Build history of the part. All positions in model axes, mm. A direction names the side the tool comes from. Give positions to 0.01 mm unless a question says otherwise; leave off trailing zeros. Write each loop counter-clockwise with the first axis right and the second up, starting at its lowest first coordinate (ties: lowest second). Pieces come first, ordered by that corner, then holes. Notation, with made-up numbers: (39, 56.5) -> (90, 56.5) arc R22 cw to (90, 76.5) -> close; hole circle Ø11 at (-14, 10.5). An arc over 180 degrees is marked (long way). One line per question, with ' | ' between items. Start each with the question number.
(1) Tool access for faces 1 (the cylindrical face through (47.882, -177.085, -476.635)), 2 (the flat face through (36, 68, -672)), 3 (the flat face through (74, 4.729, 4)): list every direction of +Z, -Z, +X, -X, +Y, -Y with a clear straight run to the whole face (end or side of a thin tool).
(2) Drill centre lines: probe 1 along Z at (x, y) = (32.5, 16.5); probe 2 along Y at (x, z) = (44, -105); probe 3 along Y at (x, z) = (63, 470.5). Where is each one in solid material? Low to high. Write a range as from..to.
(3) Pin check, flat tips, straight feed: P1, Ø6, axis at x = 110, z = -206.5, coming from the -Y side; P2, Ø7.5, axis at y = 2.5, z = 238.5, coming from the -X side. Stop position of each tip, or through.
(4) Pull direction Z, two halves, no side cores. Call faces 4 (the flat face through (156.429, 2, -2)), 5 (the flat face through (95, 31, 662)), 6 (the flat face through (55, 55, 672)), 7 (the flat face through (58, 55, -682)): released by +Z, released by -Z, zero draft, split by the parting line, or undercut.
(5) Band-saw the part on A-A, the plane y = -153.5. Give the cut face in (x, z), and give its area (3 significant figures).
from build123d import *

# Parameters (mm, degrees)
BOSS_EXTRUDE1_DEPTH      = 672
BOSS_EXTRUDE1_DEPTH_BACK = 672
SKETCH2_W                = 200
SKETCH2_H                = 116.93693015
BOSS_EXTRUDE2_DEPTH      = 10
SKETCH3_W                = 166.612048155
SKETCH3_H                = 9.263959568
BOSS_EXTRUDE4_DEPTH      = 1344
SKETCH4_W                = 200
SKETCH4_H                = 116.93693015
BOSS_EXTRUDE5_DEPTH      = 10
SKETCH5_R                = 24.75
BOSS_EXTRUDE6_DEPTH      = 350


with BuildPart() as part:
    # Sketch1 → Boss-Extrude1 (new, two sides: drawn at the far end of the back side and taken through both)
    with BuildSketch(Plane.XY.offset(-BOSS_EXTRUDE1_DEPTH_BACK)):
        with BuildLine():
            Line((156.429158375, 112.402005818), (156.429158375, 106.3293088))
            add(Edge.make_bspline(
                [(-36.718341557, -4.534924332), (65.343074275, 41.2659049), (156.429158375, 106.3293088)],
                knots=[0, 0, 0, 1, 1, 1], degree=2))
            Line((-36.718341557, -4.534924332), (-43.570841625, -4.534924332))
            add(Edge.make_bspline(
                [(-43.570841625, -4.534924332), (61.566048456, 45.124972859), (156.429158375, 112.402005818)],
                knots=[0, 0, 0, 1, 1, 1], degree=2))
        make_face()
    extrude(amount=BOSS_EXTRUDE1_DEPTH + BOSS_EXTRUDE1_DEPTH_BACK)

    # Sketch2 → Boss-Extrude2 (add)
    with BuildSketch(Plane.XY.offset(672)):
        with Locations((56.429158375, 53.933540743)):
            Rectangle(SKETCH2_W, SKETCH2_H)
    extrude(amount=-BOSS_EXTRUDE2_DEPTH)

    # Sketch3 → Boss-Extrude4 (add)
    with BuildSketch(Plane(origin=(0, 0, 662), x_dir=(-1, 0, 0), z_dir=(0, 0, -1))):
        with Locations((-73.123134298, 0.097055452)):
            Rectangle(SKETCH3_W, SKETCH3_H)
    extrude(amount=BOSS_EXTRUDE4_DEPTH)

    # Sketch4 → Boss-Extrude5 (add)
    with BuildSketch(Plane(origin=(0, 0, -682), x_dir=(-1, 0, 0), z_dir=(0, 0, -1))):
        with Locations((-56.429158375, 53.933540743)):
            Rectangle(SKETCH4_W, SKETCH4_H)
    extrude(amount=-BOSS_EXTRUDE5_DEPTH)

    # Sketch5 → Boss-Extrude6 (add)
    with BuildSketch(Plane.XZ.offset(4.534924332)):
        with Locations(Location((72.043158776, 472, 0), (0, 0, 270))):
            Circle(SKETCH5_R)
        with Locations(Location((72.043158776, -482, 0), (0, 0, 270))):
            Circle(SKETCH5_R)
    extrude(amount=BOSS_EXTRUDE6_DEPTH)


solid = part.part
Results:
1) face 1: -Y | face 2: -X, +Y | face 3: +X
2) probe 1: z = -682..-672, 662..672 | probe 2: y = -4.53..4.73, 35.64..40.89 | probe 3: y = -354.53..4.73, 46.31..51.88
3) P1: stops at y = -4.53 | P2: stops at x = -36.67
4) face 4: zero draft | face 5: undercut | face 6: released by +Z | face 7: released by -Z
5) outline: circle Ø49.5 at (72.04, -482); circle Ø49.5 at (72.04, 472) | area: 3,850 mm²
